```python
from build123d import *

# Parameters (mm, degrees)
SKETCH1_R           = 30
BOSS_EXTRUDE1_DEPTH = 80
SKETCH2_R           = 20
CUT_EXTRUDE2_DEPTH  = 77
SKETCH3_R           = 5
CUT_EXTRUDE3_DEPTH  = 20
SKETCH6_R           = 6.195708911
CUT_EXTRUDE6_DEPTH  = 40


with BuildPart() as part:
    # Sketch1 → Boss-Extrude1 (new body)
    with BuildSketch(Plane(origin=(0, 0, 0), x_dir=(1, 0, 0), z_dir=(0, 1, 0))):
        with Locations(Location((0, 0, 0), (0, 0, 270))):
            Circle(SKETCH1_R)
    extrude(amount=BOSS_EXTRUDE1_DEPTH)

    # Sketch2 → Cut-Extrude2 (cut)
    with BuildSketch(Plane(origin=(0, 80, 0), x_dir=(1, 0, 0), z_dir=(0, 1, 0))):
        with Locations(Location((0, 0, 0), (0, 0, 270))):
            Circle(SKETCH2_R)
    extrude(amount=-CUT_EXTRUDE2_DEPTH, mode=Mode.SUBTRACT)

    # Sketch3 → Cut-Extrude3 (cut)
    with BuildSketch(Plane(origin=(0, 80, 0), x_dir=(1, 0, 0), z_dir=(0, 1, 0))):
        with Locations((24.479648354, 0)):
            Circle(SKETCH3_R)
    extrude(amount=-CUT_EXTRUDE3_DEPTH, mode=Mode.SUBTRACT)

    # Sketch6 → Cut-Extrude6 (cut)
    with BuildSketch(Plane(origin=(0, 0, 0), x_dir=(0, 0, -1), z_dir=(1, 0, 0))):
        with Locations(Location((0, 60, 0), (0, 0, 180))):
            Circle(SKETCH6_R)
    extrude(amount=CUT_EXTRUDE6_DEPTH, mode=Mode.SUBTRACT)


solid = part.part
```
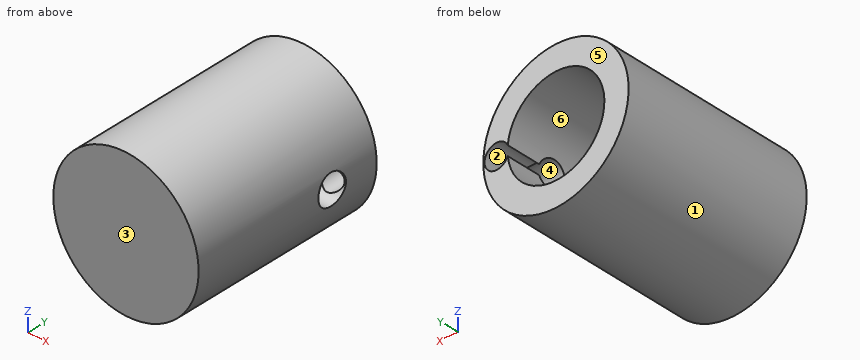
Design review of the part built by this model. Coordinates are the model's own, in mm. Face numbers are marked on the shaded views. A direction names the side the tool comes from. Round coordinates to 2 decimals unless told otherwise and drop trailing zeros. Write each loop counter-clockwise with the first axis right and the second up, starting at its lowest first coordinate (ties: lowest second). Pieces come first, ordered by that corner, then holes. Notation, with made-up numbers: (6, 76) -> (15, 76) arc R13 ccw to (15, 98) -> close; hole circle Ø6 at (70, 16). An arc over 180 degrees is marked (long way). Write item = value, one per line. Start each with the question number.
1) Wall thickness on probe 1 along X at (y, z) = (48, 0); probe 2 along Y at (x, z) = (22, 0); probe 3 along X at (y, z) = (70.5, 0): over which ranges is each line inside the solid? List them lowest first. Write a range as from..to.
2) Take a section at D-D, the plane z = -9.5. State the section outline as (x, y) points, plus the area to 3 significant figures.
3) Take a section at A-A, the plane z = 0. State the section outline as (x, y) points, plus the area to 3 significant figures.
4) Clearance check with flat-ended pins moving along their axes: pin 1 (1 mm diameter, centred on x = -19.5, y = 64, fed in from -Z); pin 2 (2 mm diameter, centred on y = 66.5, z = 11.5, fed in from +X); pin 3 (4 mm diameter, centred on y = 33, z = -2.5, fed in from -X). State where each tip first meets the part, or that it passes through.
5) Tool access review of the marked faces 5 and 6: name each direction out of +Z, -Z, +X, -X, +Y, -Y from which nothing blocks a thin tool from reaching the whole face with its end or side.
6) Take a section at C-C, the plane y = 44. State the section outline as (x, z) points.
7) Mouldability with a two-part tool opening along Z and no side actions: class the marked faces 1, 2, 3 and 4 as +Z half, -Z half, draft (parallel to the pull), parting line (faces both ways), or undercut.
8) Take a section at B-B, the plane x = 0. State the section outline as (y, z) points, plus the area to 3 significant figures.
Results list:
q1.probe_1 = -30..-20, 20..30
q1.probe_2 = 0..53.8
q1.probe_3 = -30..-20, 29.48..30
q2.outline = (-28.46, 0) -> (28.46, 0) -> (28.46, 80) -> (17.6, 80) -> (17.6, 3) -> (-17.6, 3) -> (-17.6, 80) -> (-28.46, 80) -> close
q2.area = 1,840 mm²
q3.outline = (-30, 0) -> (30, 0) -> (30, 53.8) -> (20, 53.8) -> (20, 3) -> (-20, 3) -> (-20, 80) -> (-30, 80) -> close; (29.48, 66.2) -> (30, 66.2) -> (30, 80) -> (29.48, 80) -> close
q3.area = 1,470 mm²
q4.pin_1 = -23.22
q4.pin_2 = 28.1
q4.pin_3 = -30
q5.face_5 = +Z, -Z, +X, -X, +Y
q5.face_6 = +Y
q6.outline = circle Ø60 at (0, 0); hole circle Ø40 at (0, 0)
q7.face_1 = parting line
q7.face_2 = undercut
q7.face_3 = draft
q7.face_4 = undercut
q8.outline = (0, -30) -> (80, -30) -> (80, -20) -> (3, -20) -> (3, 20) -> (80, 20) -> (80, 30) -> (0, 30) -> close
q8.area = 1,720 mm²
